Could you check a few things on this model? Use its own coordinates, in mm. Face numbers are marked on the shaded views. A direction names the side the tool comes from. Give positions to 0.01 mm unless a question says otherwise; leave off trailing zeros. Loops run counter-clockwise (first coordinate to the right, second up) from the corner with the lowest first, then second, coordinate; pieces in that order, holes last. Notation, with made-up numbers: M 7.5,-13.5 L 18.5,-13.5 A30 cw 18.5,9.5 Z; hole C 36,-29.5 d11. An arc over 180 degrees is marked long. Return JSON: item names as keys, results as strings. Group by question number.
1. If we section it at D-D (z = 22): Write out the boundary of the cut face in (x, y), plus the area to 3 significant figures.
2. If we section it at B-B (z = -3): Write out the boundary of the cut face in (x, y), plus the area to 3 significant figures.
3. If we mould it in two halves opening along X, with no side actions, what happens to the marked faces 1, 2 and 3? For each: +X half, -X half, draft (parallel to the pull), parting line (faces both ways), or undercut.
4. If we section it at C-C (y = -0.75): Write out the boundary of the cut face in (x, z) (3 decimals).
5. For pin 1 (1.1 mm diameter, centred on x = 0, z = 29.5, fed in from -Y) (3 decimals); pin 2 (4 mm diameter, centred on y = 0.5, z = 10, fed in from -X); pin 3 (1.5 mm diameter, centred on y = -1, z = 26.5, fed in from -X) (3 decimals), each with a flat end and sliding along its axis, tell me the tip position at first contact or that it passes through.
6. Please list where these lines run through material, in increasing order: line 1 (Y direction, x = 0, z = -1.45); line 2 (Z direction, x = -2.25, y = 8); line 3 (Y direction, x = 8.5, z = 28) (3 decimals).
7. If we section it at A-A (x = -4.75): Write out the boundary of the cut face in (y, z) (3 decimals).
8. For the marked faces 4, 5, 6 and 7, which set-ups out of +Z, -Z, +X, -X, +Y, -Y let a thin tool reach every point of the face, with its end or its side?
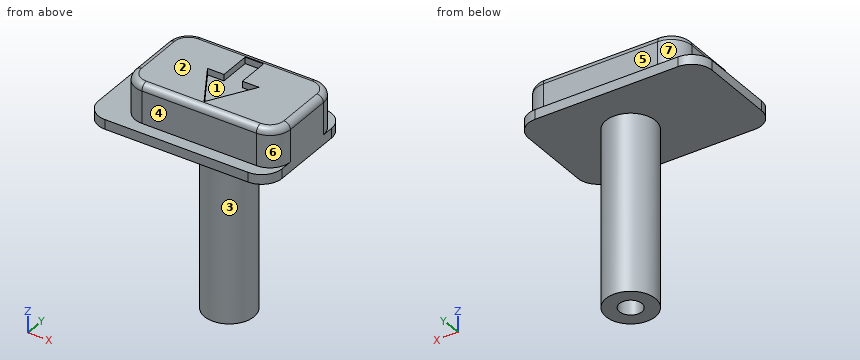
Autodesk Inventor part; units mm, degrees
ref_plane "YZ Plane" through (0, 0, 0) normal (1, 0, 0) x (0, 1, 0)
ref_plane "XZ Plane" through (0, 0, 0) normal (0, 1, 0) x (-1, 0, 0)
ref_plane "XY Plane" through (0, 0, 0) normal (0, 0, 1) x (1, 0, 0)
sketch "Sketch1" plane through (0, 0, 0) normal (0, 0, 1) x (1, 0, 0)
  circle A0 centre (0, 0) radius 1.75
  circle A1 centre (0, 0) radius 3.85
  point P0 (0, 0)
extrude "Extrusion1" add sketch "Sketch1" against normal blind 5
sketch "Sketch2" plane through (0, 0, 0) normal (0, 0, 1) x (1, 0, 0)
  point P0 (0, 0)
sketch "Sketch3" plane through (0, 0, 0) normal (0, 0, 1) x (1, 0, 0)
  circle A0 centre (0, 0) radius 3.85
extrude "Extrusion2" add sketch "Sketch3" along normal blind 22.5
sketch "Sketch4" plane through (0, 0, 22.5) normal (0, 0, 1) x (1, 0, 0)
  line L0 (12.065, -6.985) -> (-12.065, -6.985)
  line L1 (-12.065, -6.985) -> (-12.065, 6.985)
  line L2 (-12.065, 6.985) -> (12.065, 6.985)
  line L3 (12.065, 6.985) -> (12.065, -6.985)
  circle A0 centre (0, 0) radius 1.85
  line L4 (12.065, -6.985) -> (-12.065, 6.985) construction
  line L5 (-12.065, -6.985) -> (12.065, 6.985) construction
  line L6 (12.065, 12.065) -> (-12.065, 12.065) construction
  line L7 (-12.065, 12.065) -> (-12.065, 26.035) construction
  line L8 (-12.065, 26.035) -> (12.065, 26.035) construction
  line L9 (12.065, 26.035) -> (12.065, 12.065) construction
  line L10 (12.065, 12.065) -> (-12.065, 26.035) construction
  line L11 (-12.065, 12.065) -> (12.065, 26.035) construction
  line L12 (12.065, -8.89) -> (-16.51, -8.89)
  line L13 (-16.51, -8.89) -> (-16.51, 8.89)
  line L14 (-16.51, 8.89) -> (12.065, 8.89)
  line L15 (16.51, -8.89) -> (-16.51, 8.89) construction
  line L16 (-16.51, -8.89) -> (12.065, 6.4965) construction
  line L17 (12.065, -8.89) -> (12.065, 8.89)
  point P0 (0, 0)
  point P1 (0, 19.05)
  dimension "d6" = 24.13
  dimension "d7" = 13.97
  dimension "d10" = 19.05
  dimension "d16" = 17.78
extrude "Extrusion3" add sketch "Sketch4" along normal blind 1.5 contours L17 L12 L13 L14 L2 L1 L0 | L0 L1 L2 L3 | A0
extrude "Extrusion4" add sketch "Sketch4" along normal blind 7.5 contours L0 L1 L2 L3 | A0
fillet "Fillet1" radius 3.175 8 edges at (-12.065, 6.985, 27) (12.065, 6.985, 27) (12.065, -6.985, 27) (-12.065, -6.985, 27) (-16.51, -8.89, 23.25) (12.065, 8.89, 23.25) (-16.51, 8.89, 23.25) (12.065, -8.89, 23.25)
sketch "Sketch5" plane through (0, 0, 30) normal (0, 0, 1) x (1, 0, 0)
  line L0 (0, -5.8462) -> (3.9945, 0.9035)
  line L1 (-3.9945, 0.9035) -> (0, -5.8462)
  line L2 (-1.4311, 0.9035) -> (-1.4311, 5.8047)
  line L3 (-1.4311, 5.8047) -> (1.4311, 5.8047)
  line L4 (1.4311, 5.8047) -> (1.4311, 0.9035)
  line L5 (-8.89, -6.985) -> (8.89, -6.985)
  arc A0 (-8.89, 6.985) -> (-12.065, 3.81) centre (-8.89, 3.81) ccw
  line L6 (8.89, 6.985) -> (-8.89, 6.985)
  arc A1 (12.065, 3.81) -> (8.89, 6.985) centre (8.89, 3.81) ccw
  arc A2 (8.89, -6.985) -> (12.065, -3.81) centre (8.89, -3.81) ccw
  line L7 (12.065, -3.81) -> (12.065, 3.81)
  arc A3 (-12.065, -3.81) -> (-8.89, -6.985) centre (-8.89, -3.81) ccw
  line L8 (-12.065, 3.81) -> (-12.065, -3.81)
  line L9 (3.9945, 0.9035) -> (1.4311, 0.9035)
  line L10 (-1.4311, 0.9035) -> (-3.9945, 0.9035)
  point P0 (0, 0)
  point P1 (0, 0.9035)
  point P2 (0, -6.985)
emboss "Emboss1" sketch "Sketch5" operation cut depth 1 direction (0, 0, -1) contours L1 L10 L2 L3 L4 L9 L0
fillet "Fillet2" radius 1 8 edges at (-11.1351, 6.0551, 30) (-12.065, 0, 30) (-11.1351, -6.0551, 30) (0, -6.985, 30) (11.1351, -6.0551, 30) (12.065, 0, 30) (11.1351, 6.0551, 30) (0, 6.985, 30)
properties part number "Button Cover"
Answer:
{
 "1": {"outline": "C 0,0 d7.7", "area": "46.6 mm²"},
 "2": {"outline": "C 0,0 d7.7; hole C 0,0 d3.5", "area": "36.9 mm²"},
 "3": {"face 1": "undercut", "face 2": "draft", "face 3": "parting line"},
 "4": {"outline": "M -16.51,22.5 L -3.776,22.5 L -3.776,-5 L -1.581,-5 L -1.581,0 L 1.581,0 L 1.581,-5 L 3.776,-5 L 3.776,22.5 L 12.065,22.5 L 12.065,29 A1 ccw 11.065,30 L 3.016,30 L 3.016,29 L -3.016,29 L -3.016,30 L -11.065,30 A1 ccw -12.065,29 L -12.065,24 L -16.51,24 Z"},
 "5": {"pin 1": "stops at y = -6.985", "pin 2": "stops at x = -3.85", "pin 3": "stops at x = -12.065"},
 "6": {"line 1": "y = -3.85 to -1.75, 1.75 to 3.85", "line 2": "z = 22.5 to 24", "line 3": "y = -6.985 to 6.985"},
 "7": {"outline": "M -8.89,22.5 L 8.89,22.5 L 8.89,24 L 6.985,24 L 6.985,29 A1 ccw 5.985,30 L -5.985,30 A1 ccw -6.985,29 L -6.985,24 L -8.89,24 Z"},
 "8": {"face 4": "+Z, +X, -X, -Y", "face 5": "+Z, +X, -X, +Y", "face 6": "+Z, +X, -Y", "face 7": "+Z, -X, +Y"}
}
